Could you check a few things on this model? Use its own coordinates, in mm. Coordinates: 2 decimals unless noted, no trailing zeros. Write each loop counter-clockwise with the first axis right and the second up, starting at its lowest first coordinate (ties: lowest second). Pieces come first, ordered by that corner, then holes. Notation, with made-up numbers: M -36,-16 L 21,-16 A16 ccw 21,9 Z; hole C 60.5,17 d6. An arc over 180 degrees is marked long. Answer as CSV lines item,"result". Start each with the question number.
Item 1: Suppose I cut it at A-A, the plane z = 0.25. Write out the boundary of the cut face in (x, y), and give its area (3 significant figures).
Item 2: Suppose I cut it at B-B, the plane y = -72. Write out the boundary of the cut face in (x, z), and give its area (3 significant figures).
Item 3: I'm going to push flat-ended pins straight in: P1, Ø2.5, axis at x = -60.68, y = 119.31, coming from the -Z side; P2, Ø6.5, axis at x = 59, y = 119.31, coming from the +Z side. Where does each tip first touch, or does it pass through?
Item 4: If I drill on line 1 along X through (y, z) = (-84.5, 0.2); line 2 along X through (y, z) = (-99.5, 1); line 3 along Y through (x, z) = (-76, 0.2), over which ranges is the centre line in solid material (lowest first)? Write a range as [from, to].
Item 5: Suppose I cut it at C-C, the plane x = 69.5. Write out the boundary of the cut face in (y, z), and give its area (3 significant figures).
```python
from build123d import *

# Parameters (mm, degrees)
RESSALTO_EXTRUS_O1_DEPTH = 1.5
CORTE_EXTRUS_O1_REACH    = 3.5
ESBO_O2_R                = 2.1


with BuildPart() as part:
    # Esboço1 → Ressalto-extrusão1 (new body)
    with BuildSketch(Plane.XY):
        Polygon((55.321046002, 133.809611411), (-57.006999458, 133.809611411), (-95.842976728, 87.526695978), (-95.842976728, 22.140182404), (-50.842976728, -31.488729263), (-50.842976728, -135.082673958), (-49.522853837, -136.190388589), (47.836900381, -136.190388589), (49.157023272, -135.082673958), (49.157023272, -31.488729263), (94.157023272, 22.140182404), (94.157023272, 87.526695978), align=None)
    extrude(amount=RESSALTO_EXTRUS_O1_DEPTH)

    # Esboço2 → Corte-extrusão1 (cut, up to next)
    with BuildSketch(Plane.XY.offset(1.5), mode=Mode.PRIVATE) as corte_extrus_o1_sk1:
        with Locations((-60.684933322, 119.314215641)):
            Circle(ESBO_O2_R)
    corte_extrus_o1_tool1 = extrude(corte_extrus_o1_sk1.sketch, amount=-CORTE_EXTRUS_O1_REACH, mode=Mode.PRIVATE) & part.part
    add(corte_extrus_o1_tool1.solids().sort_by_distance((-60.684933, 119.314216, 1.5))[0], mode=Mode.SUBTRACT)
    # Esboço2 → Corte-extrusão1 (cut, up to next)
    with BuildSketch(Plane.XY.offset(1.5), mode=Mode.PRIVATE) as corte_extrus_o1_sk2:
        with Locations((-44.342976728, -101.030388589)):
            Circle(ESBO_O2_R)
    corte_extrus_o1_tool2 = extrude(corte_extrus_o1_sk2.sketch, amount=-CORTE_EXTRUS_O1_REACH, mode=Mode.PRIVATE) & part.part
    add(corte_extrus_o1_tool2.solids().sort_by_distance((-44.342977, -101.030389, 1.5))[0], mode=Mode.SUBTRACT)
    # Esboço2 → Corte-extrusão1 (cut, up to next)
    with BuildSketch(Plane.XY.offset(1.5), mode=Mode.PRIVATE) as corte_extrus_o1_sk3:
        with Locations((42.657023272, -101.030388589)):
            Circle(ESBO_O2_R)
    corte_extrus_o1_tool3 = extrude(corte_extrus_o1_sk3.sketch, amount=-CORTE_EXTRUS_O1_REACH, mode=Mode.PRIVATE) & part.part
    add(corte_extrus_o1_tool3.solids().sort_by_distance((42.657023, -101.030389, 1.5))[0], mode=Mode.SUBTRACT)
    # Esboço2 → Corte-extrusão1 (cut, up to next)
    with BuildSketch(Plane.XY.offset(1.5), mode=Mode.PRIVATE) as corte_extrus_o1_sk4:
        with Locations((58.998979866, 119.314215641)):
            Circle(ESBO_O2_R)
    corte_extrus_o1_tool4 = extrude(corte_extrus_o1_sk4.sketch, amount=-CORTE_EXTRUS_O1_REACH, mode=Mode.PRIVATE) & part.part
    add(corte_extrus_o1_tool4.solids().sort_by_distance((58.99898, 119.314216, 1.5))[0], mode=Mode.SUBTRACT)
    # Esboço2 → Corte-extrusão1 (cut, up to next)
    with BuildSketch(Plane.XY.offset(1.5), mode=Mode.PRIVATE) as corte_extrus_o1_sk5:
        with Locations((-44.342976728, -51.190388589)):
            Circle(ESBO_O2_R)
    corte_extrus_o1_tool5 = extrude(corte_extrus_o1_sk5.sketch, amount=-CORTE_EXTRUS_O1_REACH, mode=Mode.PRIVATE) & part.part
    add(corte_extrus_o1_tool5.solids().sort_by_distance((-44.342977, -51.190389, 1.5))[0], mode=Mode.SUBTRACT)


solid = part.part
```
Ans:
1,outline,"M -95.84,22.14 L -50.84,-31.49 L -50.84,-135.08 L -49.52,-136.19 L 47.84,-136.19 L 49.16,-135.08 L 49.16,-31.49 L 94.16,22.14 L 94.16,87.53 L 55.32,133.81 L -57.01,133.81 L -95.84,87.53 Z; hole C -60.68,119.31 d4.2; hole C -44.34,-101.03 d4.2; hole C -44.34,-51.19 d4.2; hole C 42.66,-101.03 d4.2; hole C 59,119.31 d4.2"
1,area,"37,600 mm^2"
2,outline,"M -50.84,0 L 49.16,0 L 49.16,1.5 L -50.84,1.5 Z"
2,area,"150 mm^2"
3,P1,"passes through"
3,P2,"stops at z = 1.5"
4,line 1,"x = [-50.84, 49.16]"
4,line 2,"x = [-50.84, -45.78], [-42.9, 41.22], [44.1, 49.16]"
4,line 3,"y = [-1.51, 111.17]"
5,outline,"M -7.24,0 L 116.91,0 L 116.91,1.5 L -7.24,1.5 Z"
5,area,"186 mm^2"
